For this review, take the finished solid that the model builds, in its own axes (mm). Face numbers are marked on the shaded views. A direction names the side the tool comes from. Round coordinates to 2 decimals unless told otherwise and drop trailing zeros. Write each loop counter-clockwise with the first axis right and the second up, starting at its lowest first coordinate (ties: lowest second). Pieces come first, ordered by that corner, then holes. Notation, with made-up numbers: (36.25, 86.25) - (72.25, 86.25) arc R30 cw to (72.25, 116.25) - close; hole circle Ø8 at (84.5, 5.5). An arc over 180 degrees is marked (long way). One line per item, written item: value. Start each with the question number.
Q1. Tool access review of the marked faces 4, 5 and 6: name each direction out of +Z, -Z, +X, -X, +Y, -Y from which nothing blocks a thin tool from reaching the whole face with its end or side.
Q2. Clearance check with flat-ended pins moving along their axes: pin 1 Ø2 at (x, z) = (3.5, 13.5) entering from +Y; pin 2 Ø5.5 at (y, z) = (0, 23.5) entering from +X; pin 3 Ø3.5 at (x, y) = (0, 0) entering from -Z. State where each tip first meets the part, or that it passes through.
Q3. For probe 1 along Y at (x, z) = (0, 3.5); probe 2 along X at (y, z) = (-1.5, 5); probe 3 along Y at (x, z) = (-1, -0.5), list the stretches that pass through material, from the lowest coordinate up.
Q4. Add section A-A on z = 27. Write out the cut boundary in (x, y).
Q5. Add section B-B on z = 11. Write out the cut boundary in (x, y).
Q6. Mouldability with a two-part tool opening along X and no side actions: class the marked faces 1, 2 and 3 as +X half, -X half, draft (parallel to the pull), parting line (faces both ways), or undercut.
```python
from build123d import *

# Parameters (mm, degrees)
ESQUISSE1_R             = 6
BOSS_EXTRU_1_DEPTH      = 12
ESQUISSE2_R             = 5
BOSS_EXTRU_2_DEPTH      = 9
ESQUISSE3_R             = 7.25
BOSS_EXTRU_3_DEPTH      = 2.5
ESQUISSE4_R             = 2
ENL_V_MAT_EXTRU_1_DEPTH = 20
ESQUISSE9_R             = 2.1
ENL_V_MAT_EXTRU_4_DEPTH = 5.5
ESQUISSE6_R             = 4.25
ESQUISSE6_R_2           = 2.5
ENL_V_MAT_EXTRU_2_DEPTH = 10
CHANFREIN1_SIZE         = 0.5
CHANFREIN2_SIZE         = 0.2
BOSS_EXTRU_4_DEPTH      = 0.4
BOSS_EXTRU_4_DEPTH_BACK = 0.4
ESQUISSE8_R             = 0.65
CHANFREIN3_SIZE         = 1
CHANFREIN3_SIZE2        = 0.267949192
CHANFREIN4_SIZE         = 1
CHANFREIN4_SIZE2        = 0.267949192


with BuildPart() as part:
    # Esquisse1 → Boss.-Extru.1 (new body)
    with BuildSketch(Plane.XY):
        Circle(ESQUISSE1_R)
    extrude(amount=BOSS_EXTRU_1_DEPTH)

    # Esquisse2 → Boss.-Extru.2 (add)
    with BuildSketch(Plane.XY.offset(12)):
        Circle(ESQUISSE2_R)
    extrude(amount=BOSS_EXTRU_2_DEPTH)

    # Esquisse3 → Boss.-Extru.3 (add)
    with BuildSketch(Plane(origin=(0, 0, 0), x_dir=(-1, 0, 0), z_dir=(0, 0, -1))):
        Circle(ESQUISSE3_R)
    extrude(amount=BOSS_EXTRU_3_DEPTH)

    # Esquisse4 → Enlèv. mat.-Extru.1 (cut)
    with BuildSketch(Plane(origin=(0, 0, -2.5), x_dir=(-1, 0, 0), z_dir=(0, 0, -1))):
        Circle(ESQUISSE4_R)
    extrude(amount=-ENL_V_MAT_EXTRU_1_DEPTH, mode=Mode.SUBTRACT)

    # Esquisse9 → Enlèv. mat.-Extru.4 (cut)
    with BuildSketch(Plane(origin=(0, 0, -2.5), x_dir=(-1, 0, 0), z_dir=(0, 0, -1))):
        Circle(ESQUISSE9_R)
    extrude(amount=-ENL_V_MAT_EXTRU_4_DEPTH, mode=Mode.SUBTRACT)

    # Esquisse6 → Enlèv. mat.-Extru.2 (cut)
    with BuildSketch(Plane(origin=(0, 0, -2.5), x_dir=(-1, 0, 0), z_dir=(0, 0, -1))):
        Circle(ESQUISSE6_R)
        Circle(ESQUISSE6_R_2, mode=Mode.SUBTRACT)
    extrude(amount=-ENL_V_MAT_EXTRU_2_DEPTH, mode=Mode.SUBTRACT)

    # Chanfrein1
    chanfrein1_edges = [part.edges().sort_by_distance(p)[0] for p in [
        (4.25, 0, -2.5),
        (-6, 0, 12),
        (-5, 0, 21),
        (7.25, 0, -2.5),
    ]]
    chamfer(chanfrein1_edges, length=CHANFREIN1_SIZE)

    # Chanfrein2
    chanfrein2_edges = [part.edges().sort_by_distance(p)[0] for p in [
        (2.5, 0, -2.5),
    ]]
    chamfer(chanfrein2_edges, length=CHANFREIN2_SIZE)

    # Esquisse8 → Boss.-Extru.4 (add, two sides: drawn at the far end of the back side and taken through both)
    with BuildSketch(Plane(origin=(0, 0, 0), x_dir=(0, 0, -1), z_dir=(1, 0, 0)).offset(-BOSS_EXTRU_4_DEPTH_BACK)):
        Polygon((-21, -2.4), (-28.5, -2.4), (-29.5, -1.4), (-29.5, 1.4), (-28.5, 2.4), (-21, 2.4), align=None)
        with Locations((-27, 0)):
            Circle(ESQUISSE8_R, mode=Mode.SUBTRACT)
    extrude(amount=BOSS_EXTRU_4_DEPTH + BOSS_EXTRU_4_DEPTH_BACK)

    # Chanfrein3
    chanfrein3_edges = [part.edges().sort_by_distance(p)[0] for p in [
        (0.4, 0, 29.5),
    ]]
    chanfrein3_side = [part.faces().sort_by_distance(p)[0] for p in [
        (0.4, 0, 25.087820443),
    ]]
    chamfer(chanfrein3_edges, length=CHANFREIN3_SIZE, length2=CHANFREIN3_SIZE2, reference=chanfrein3_side[0])

    # Chanfrein4
    chanfrein4_edges = [part.edges().sort_by_distance(p)[0] for p in [
        (-0.4, 0, 29.5),
    ]]
    chanfrein4_side = [part.faces().sort_by_distance(p)[0] for p in [
        (-0.4, 0, 25.087820443),
    ]]
    chamfer(chanfrein4_edges, length=CHANFREIN4_SIZE, length2=CHANFREIN4_SIZE2, reference=chanfrein4_side[0])


solid = part.part
```
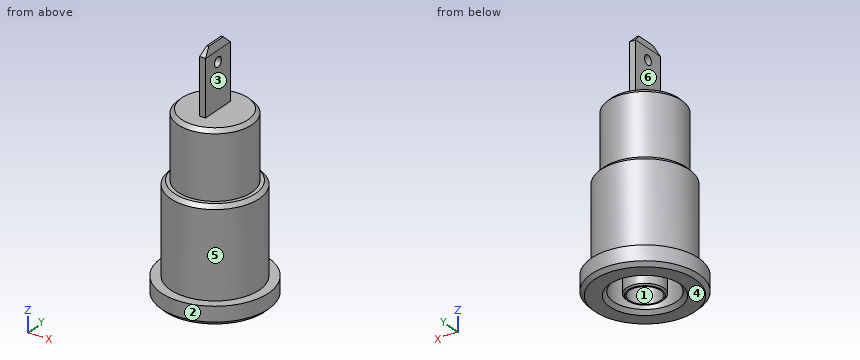
Result set:
1. face 4: -Z, +X, -X, +Y, -Y
1. face 5: +Z
1. face 6: +Z, -X, +Y, -Y
2. pin 1: stops at y = 4.33
2. pin 2: stops at x = 4.75
2. pin 3: stops at z = 17.5
3. probe 1: y = -6 to -4.25, -2.5 to -2, 2 to 2.5, 4.25 to 6
3. probe 2: x = -5.81 to -3.98, -2 to -1.32, 1.32 to 2, 3.98 to 5.81
3. probe 3: y = -7.18 to -4.13, -2.29 to -1.85, 1.85 to 2.29, 4.13 to 7.18
4. outline: (-0.4, -2.4) - (0.4, -2.4) - (0.4, -0.65) - (-0.4, -0.65) - close; (-0.4, 0.65) - (0.4, 0.65) - (0.4, 2.4) - (-0.4, 2.4) - close
5. outline: circle Ø12 at (0, 0); hole circle Ø4 at (0, 0)
6. face 1: undercut
6. face 2: parting line
6. face 3: +X half
